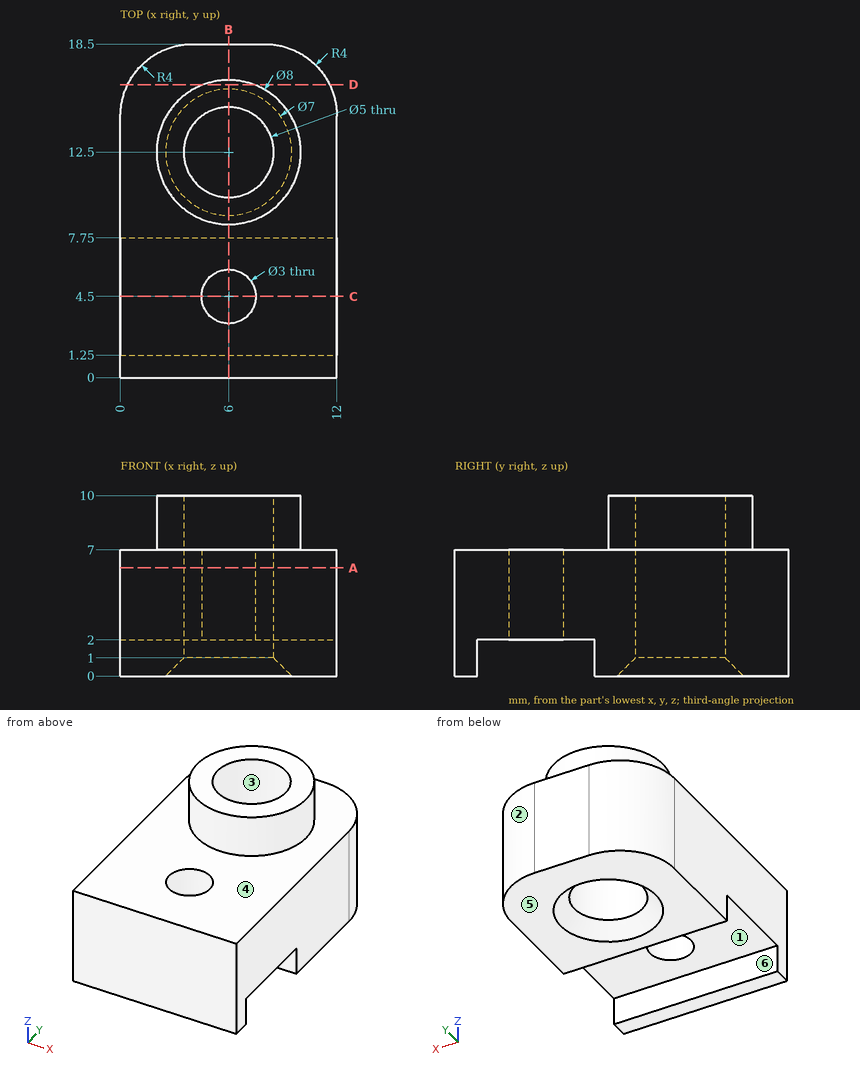
For this review, use the dimensioned drawing (mm, ordinates from the lowest corner) and the shaded views. A direction names the side the tool comes from. Coordinates: 2 decimals unless noted, no trailing zeros. Loops run counter-clockwise (first coordinate to the right, second up) from the corner with the lowest first, then second, coordinate; pieces in that order, holes last.
1. Add section B-B, the plane x = 6. Give the boundary of the cut face in (y, z), then the cut area to 3 significant figures.
2. Add section D-D, the plane y = 16.25. Give the boundary of the cut face in (x, z), then the cut area to 3 significant figures.
3. For the marked faces 4, 5 and 6, list the 3-axis set-ups (+Z, -Z, +X, -X, +Y, -Y) from which the entire face can be reached by the end or side of a thin tool; tool diameter is ignored.
4. Add section C-C, the plane y = 4.5. Give the boundary of the cut face in (x, z).
5. Mouldability with a two-part tool opening along X and no side actions: class the marked faces 1, 2 and 3 as +X half, -X half, draft (parallel to the pull), parting line (faces both ways), or undercut.
6. For line 1 (Y direction, x = 6, z = 4.5); line 2 (X direction, y = 4.5, z = 3.4); line 3 (Z direction, x = 4.5, y = 5.25), list the stretches that pass through material, from the lowest coordinate up.
7. Insertion check: P1, Ø1, axis at x = 5.5, z = 1.5, coming from the -Y side; P2, Ø0.6, axis at x = 3, z = 1.5, coming from the +Y side; P3, Ø3, axis at x = 3.5, y = 5, coming from the -Z side; P4, Ø6, axis at x = 6, y = 12.5, coming from the -Z side. Each pin has a flat end and moves straight along its axis. Give the tip position at first contact, or say it passes through.
8. Add section A-A, the plane z = 6. Give the boundary of the cut face in (x, y), then the cut area to 3 significant figures.
Result:
1. outline: (0, 0) - (1.25, 0) - (1.25, 2) - (3, 2) - (3, 7) - (0, 7) - close; (6, 2) - (7.75, 2) - (7.75, 0) - (9, 0) - (10, 1) - (10, 10) - (8.5, 10) - (8.5, 7) - (6, 7) - close; (15, 1) - (16, 0) - (18.5, 0) - (18.5, 7) - (16.5, 7) - (16.5, 10) - (15, 10) - close
1. area: 74.5 mm2
2. outline: (0.4, 0) - (11.6, 0) - (11.6, 7) - (7.39, 7) - (7.39, 10) - (4.61, 10) - (4.61, 7) - (0.4, 7) - close
2. area: 86.7 mm2
3. face 4: +Z
3. face 5: -Z, +X, -X, +Y, -Y
3. face 6: -Z, +X, -X
4. outline: (0, 2) - (4.5, 2) - (4.5, 7) - (0, 7) - close; (7.5, 2) - (12, 2) - (12, 7) - (7.5, 7) - close
5. face 1: draft
5. face 2: +X half
5. face 3: undercut
6. line 1: y = 0 to 3, 6 to 10, 15 to 18.5
6. line 2: x = 0 to 4.5, 7.5 to 12
6. line 3: z = 2 to 7
7. P1: stops at y = 0
7. P2: stops at y = 18.44
7. P3: stops at z = 2
7. P4: stops at z = 0.5
8. outline: (0, 0) - (12, 0) - (12, 14.5) arc R4 ccw to (8, 18.5) - (4, 18.5) arc R4 ccw to (0, 14.5) - close; hole circle Ø5 at (6, 12.5); hole circle Ø3 at (6, 4.5)
8. area: 188 mm2
